Read the model definition and answer for the solid it produces. Units are mm, in the model's axes. Face numbers are marked on the shaded views. Give positions to 0.01 mm unless a question says otherwise; leave off trailing zeros. Order: outer loops, then holes, each group sorted by start corner. A loop starts at its lowest first (then second) coordinate and runs counter-clockwise, first axis right, second up. Notation, with made-up numbers: (-15.5, -8) - (32.5, -8) arc R30 cw to (32.5, 29) - close; hole circle Ø7 at (-26, 41.5). An arc over 180 degrees is marked (long way). Write item = value, one per line.
```python
from build123d import *

# Parameters (mm, degrees)
SKETCH1_W           = 50.8
SKETCH1_H           = 63.5
BOSS_EXTRUDE1_DEPTH = 6.35
SKETCH2_R           = 15.875
CUT_EXTRUDE1_DEPTH  = 13.7
SKETCH3_R           = 3.175
CUT_EXTRUDE2_DEPTH  = 12.7


with BuildPart() as part:
    # Sketch1 → Boss-Extrude1 (new body, symmetric)
    with BuildSketch(Plane(origin=(0, 0, 0), x_dir=(1, 0, 0), z_dir=(0, 1, 0))):
        with Locations((0, 6.35)):
            Rectangle(SKETCH1_W, SKETCH1_H)
    extrude(amount=BOSS_EXTRUDE1_DEPTH, both=True)

    # Sketch2 → Cut-Extrude1 (cut, through all)
    with BuildSketch(Plane(origin=(0, 6.35, 0), x_dir=(1, 0, 0), z_dir=(0, 1, 0))):
        Circle(SKETCH2_R)
    extrude(amount=-CUT_EXTRUDE1_DEPTH, mode=Mode.SUBTRACT)

    # Sketch3 → Cut-Extrude2 (cut)
    with BuildSketch(Plane(origin=(0, 0, -38.1), x_dir=(-1, 0, 0), z_dir=(0, 0, -1))):
        with Locations((-15.875, 0)):
            Circle(SKETCH3_R)
        with Locations((15.875, 0)):
            Circle(SKETCH3_R)
    extrude(amount=-CUT_EXTRUDE2_DEPTH, mode=Mode.SUBTRACT)


solid = part.part
```
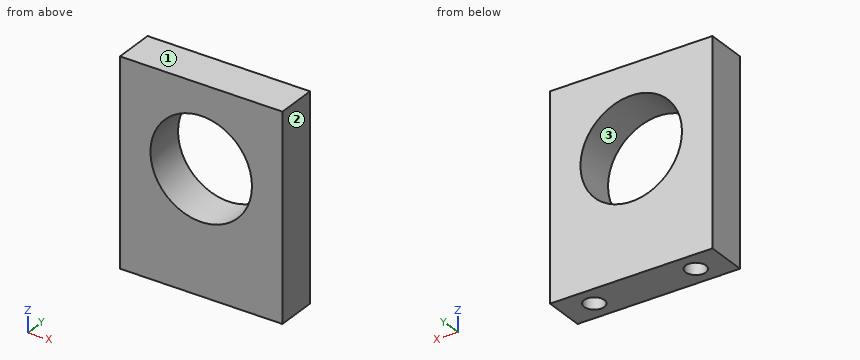
1. Section D-D (y = 4.5) is taken. Determine the outline of the cut face in (x, z) (3 decimals).
Recorded:
outline = (-25.4, -38.1) - (25.4, -38.1) - (25.4, 25.4) - (-25.4, 25.4) - close; hole circle Ø31.75 at (0, 0)
2. Section B-B (y = 0) is taken. Determine the outline of the cut face in (x, z) (3 decimals), and give its area (3 significant figures).
Recorded:
outline = (-25.4, -38.1) - (-19.05, -38.1) - (-19.05, -25.4) - (-12.7, -25.4) - (-12.7, -38.1) - (12.7, -38.1) - (12.7, -25.4) - (19.05, -25.4) - (19.05, -38.1) - (25.4, -38.1) - (25.4, 25.4) - (-25.4, 25.4) - close; hole circle Ø31.75 at (0, 0)
area = 2,270 mm^2
3. Section C-C (z = 0) is taken. Determine the outline of the cut face in (x, y) (3 decimals).
Recorded:
outline = (-25.4, -6.35) - (-15.875, -6.35) - (-15.875, 6.35) - (-25.4, 6.35) - close; (15.875, -6.35) - (25.4, -6.35) - (25.4, 6.35) - (15.875, 6.35) - close
4. Section A-A (x = 0) is taken. Determine the outline of the cut face in (y, z) (3 decimals).
Recorded:
outline = (-6.35, -38.1) - (6.35, -38.1) - (6.35, -15.875) - (-6.35, -15.875) - close; (-6.35, 15.875) - (6.35, 15.875) - (6.35, 25.4) - (-6.35, 25.4) - close
5. Straight lines are drawn through the part: L1, parallel to Z at x = 0, y = -2.5 (3 decimals); L2, parallel to X at y = -2, z = 0 (3 decimals); L3, parallel to Z at x = 7.5, y = -2. For each, find the intervals that lie inside material, in ascending order. Write a range as [from, to].
Recorded:
L1 = [-38.1, -15.875], [15.875, 25.4]
L2 = [-25.4, -15.875], [15.875, 25.4]
L3 = [-38.1, -13.99], [13.99, 25.4]
6. Determine the mould class of the marked faces 1, 2 and 3 for opening direction Z: +Z half, -Z half, draft (parallel to the pull), parting line (faces both ways), or undercut.
Recorded:
face_1 = +Z half
face_2 = draft
face_3 = undercut
7. A flat-ended cylindrical pin translates along its axis: pin 1 (3 mm diameter, centred on x = 16.5, y = -1, fed in from -Z). Find the tip coordinate at first contact, or state that the pin passes through.
Recorded:
pin_1 = -25.4
